Design review of the part built by this model. Coordinates are the model's own, in mm. A direction names the side the tool comes from. Give positions to 0.01 mm unless a question says otherwise; leave off trailing zeros. Loops run counter-clockwise (first coordinate to the right, second up) from the corner with the lowest first, then second, coordinate; pieces in that order, holes last. Notation, with made-up numbers: (72.5, -5.5) - (120.5, -5.5) arc R15 cw to (120.5, 5.5) - close; hole circle Ø8 at (-11.75, -36.5). An arc over 180 degrees is marked (long way). Put each result on its own line as item: value. Start each with the question number.
Autodesk Inventor part; units mm, degrees
ref_plane "YZ Plane" through (0, 0, 0) normal (1, 0, 0) x (0, 1, 0)
ref_plane "XZ Plane" through (0, 0, 0) normal (0, 1, 0) x (-1, 0, 0)
ref_plane "XY Plane" through (0, 0, 0) normal (0, 0, 1) x (1, 0, 0)
sketch "Sketch1" plane through (0, 0, 0) normal (0, 1, 0) x (-1, 0, 0)
  line L0 (0, 0) -> (86.36, 0)
  line L1 (86.36, 0) -> (86.36, -180.34)
  line L2 (86.36, -180.34) -> (0, -180.34)
  line L3 (0, -180.34) -> (0, 0)
  line L4 (-2.4049, 2.4049) -> (88.7649, 2.4049)
  line L5 (88.7649, 2.4049) -> (88.7649, -182.7449)
  line L6 (88.7649, -182.7449) -> (-2.4049, -182.7449)
  line L7 (-2.4049, -182.7449) -> (-2.4049, 2.4049)
  line L8 (-8.7549, 8.7549) -> (95.1149, 8.7549)
  line L9 (95.1149, 8.7549) -> (95.1149, -189.0949)
  line L10 (95.1149, -189.0949) -> (-8.7549, -189.0949)
  line L11 (-8.7549, -189.0949) -> (-8.7549, 8.7549)
  line L12 (86.36, 0) -> (86.36, 48.8454)
  line L13 (86.36, 48.8454) -> (86.36, -245.5667)
  line L14 (86.36, 8.7549) -> (73.66, 8.7549)
  line L15 (73.66, 8.7549) -> (73.66, 34.1549)
  line L16 (73.66, 34.1549) -> (86.36, 34.1549)
  line L17 (86.36, 34.1549) -> (86.36, 8.7549)
  line L18 (86.36, -189.0949) -> (73.66, -189.0949)
  line L19 (73.66, -189.0949) -> (73.66, -214.4949)
  line L20 (73.66, -214.4949) -> (86.36, -214.4949)
  line L21 (86.36, -214.4949) -> (86.36, -189.0949)
  point P0 (86.36, 34.1549)
  point P1 (73.66, 8.7549)
  point P2 (73.66, -189.0949)
  point P3 (86.36, -214.4949)
  point P4 (86.36, -182.7449)
  point P5 (86.36, 2.4049)
  dimension "d0" = 86.36
  dimension "d1" = 180.34
  dimension "d2" = 6.35
  dimension "d3" = 12.7
  dimension "d4" = 25.4
  dimension "d5" = 12.7
  dimension "d6" = 25.4
extrude "Extrusion1" add sketch "Sketch1" along normal blind 25.4 contours L4 L7 L6 L13 L10 L11 L8 L12 | L8 L15 L16 L12 | L13 L20 L19 L10
fillet "Fillet1" radius 3.175 4 edges at (8.7549, 12.7, 8.7549) (8.7549, 12.7, -189.0949) (-73.66, 12.7, 8.7549) (-73.66, 12.7, -189.0949)
fillet "Fillet2" radius 12.7 4 edges at (-80.01, 25.4, 34.1549) (-80.01, 0, 34.1549) (-80.01, 25.4, -214.4949) (-80.01, 0, -214.4949)
sketch "Sketch2" plane through (-73.66, 0, -192.2699) normal (1, 0, 0) x (0, 0, -1)
  arc A0 (-213.7248, 25.4) -> (-213.7248, 0) centre (-213.7248, 12.7) ccw
  line L0 (-213.7248, 0) -> (-204.1998, 0)
  line L1 (-204.1998, 25.4) -> (-204.1998, 0)
  line L2 (-213.7248, 25.4) -> (-204.1998, 25.4)
  arc A1 (9.525, 0) -> (9.525, 25.4) centre (9.525, 12.7) ccw
  line L3 (0, 25.4) -> (9.525, 25.4)
  line L4 (0, 0) -> (0, 25.4)
  line L5 (0, 0) -> (9.525, 0)
  circle A2 centre (-213.7248, 12.7) radius 3.175
  circle A3 centre (9.525, 12.7) radius 3.175
  point P0 (-192.2699, 0)
  dimension "d11" = 6.35
  dimension "d12" = 6.35
extrude "Extrusion2" cut sketch "Sketch2" against normal blind 25.4 contours A2 | A3
sketch "Sketch3" plane through (8.7549, 0, 5.5799) normal (1, 0, 0) x (0, 0, -1)
  line L0 (0, 25.4) -> (191.4998, 25.4)
  line L1 (95.7499, 25.4) -> (95.7499, 0)
  line L2 (188.3248, 0) -> (3.175, 0)
  line L3 (83.0499, 25.4) -> (83.0499, 0)
  point P0 (5.5799, 0)
  point P1 (83.0499, 0)
  dimension "d15" = 12.7
extrude "Extrusion3" add sketch "Sketch3" along normal blind 25.4
sketch "Sketch4" plane through (8.7549, 0, -185.9199) normal (1, 0, 0) x (0, 0, -1)
  line L0 (-3.175, 25.4) -> (-188.3248, 25.4)
  line L1 (-95.7499, 25.4) -> (115.4033, 25.4)
  line L2 (115.4033, 25.4) -> (115.4033, -38.5479)
  line L3 (115.4033, -38.5479) -> (-95.7499, -38.5479)
  line L4 (-95.7499, -38.5479) -> (-95.7499, 25.4)
  point P0 (-185.9199, 0)
  point P1 (-3.175, 25.4)
extrude "Extrusion4" cut sketch "Sketch4" along normal through all both and the other way through all
fillet "Fillet3" radius 12.7 2 edges at (34.1549, 25.4, -83.82) (34.1549, 0, -83.82)
fillet "Fillet4" radius 3.175 1 edges at (8.7549, 12.7, -77.47)
sketch "Sketch5" plane through (21.4549, 12.7, -77.47) normal (0, 0, 1) x (1, 0, 0)
  arc A0 (0, -12.7) -> (0, 12.7) centre (0, 0) ccw
  circle A1 centre (0, 0) radius 3.175
  point P0 (-21.4549, -12.7)
  dimension "d22" = 6.35
extrude "Extrusion5" cut sketch "Sketch5" against normal blind 25.4
properties part number "Battery mount top" material "Rubber, Silicone"
Item 1: Consider section C-C (y = 2.75). State the section outline as (x, z) points (3 decimals).
Item 2: Consider section B-B (x = 23). State the section outline as (y, z) points.
Item 3: Consider section D-D (z = -63). State the section outline as (x, y) points, plus the area to 3 significant figures.
Item 4: For P1, Ø1, axis at x = -16.5, y = 3.5, coming from the +Z side; P2, Ø8, axis at x = -20.5, z = 11.5, coming from the -Y side; P3, Ø7.5, axis at y = 8, z = -65.5, coming from the -X side; P4, Ø7.5, axis at x = -63, y = 7.5, coming from the -Z side, all flat-tipped, find the tip position at first contact; note any pin that passes through.
Item 5: Machinability: for faces 4 (the flat face through (2.405, 13, -45)), 5 (the flat face through (-32, 13, 8.755)), 6 (the flat face through (18, 13, -90.17)), which of the approach directions +Z, -Z, +X, -X, +Y, -Y give a long, thin tool a straight path to every point of the face, cutting with its end or side? Answer none if there is none.
Item 6: Mouldability with a two-part tool opening along X and no side actions: class faces 1 (the flat face through (-41, 13, 2.405)), 2 (the cylindrical face through (30.336, 21.779, -83.909)), 3 (the cylindrical face through (18.283, 12.84, -83.731)) as pulls with the +X half, pulls with the -X half, needs draft (parallel to the pull), parting line crosses it, or undercut.
Item 7: For L1, parallel to Z at x = -43.5, y = 12.5; L2, parallel to X at y = 5, z = 22.5, list the stretches that pass through material, from the lowest coordinate up. Write a range as from..to.
Geometry says:
1. outline: (-86.36, 2.405) - (2.405, 2.405) - (2.405, -90.17) - (29.347, -90.17) - (29.347, -77.47) - (11.93, -77.47) arc R3.175 cw to (8.755, -74.295) - (8.755, 5.58) arc R3.175 ccw to (5.58, 8.755) - (-70.485, 8.755) arc R3.175 cw to (-73.66, 11.93) - (-73.66, 29.347) - (-86.36, 29.347) - close
2. outline: (0.09, -90.17) - (9.93, -90.17) - (9.93, -77.47) - (0.09, -77.47) - close; (15.47, -90.17) - (25.31, -90.17) - (25.31, -77.47) - (15.47, -77.47) - close
3. outline: (2.4, 0) - (8.75, 0) - (8.75, 25.4) - (2.4, 25.4) - close
3. area: 161 mm2
4. P1: stops at z = 8.75
4. P2: stops at y = 0
4. P3: stops at x = 2.4
4. P4: stops at z = 2.4
5. face 4: -Z, -X, +Y, -Y
5. face 5: +Z, +X, +Y, -Y
5. face 6: -Z, +X, -X, +Y, -Y
6. face 1: needs draft
6. face 2: pulls with the +X half
6. face 3: undercut
7. L1: z = 2.4..8.75
7. L2: x = -86.36..-73.66
